Can you work these out from the drawing? Everything is in mm from the part's minimum corner. Give positions to 0.01 mm unless a question says otherwise; leave off trailing zeros. Write each loop counter-clockwise with the first axis right and the second up, starting at its lowest first coordinate (ties: lowest second). Pieces come first, ordered by that corner, then holes. Notation, with made-up numbers: (45, -37) - (89, -37) arc R19 ccw to (89, -7) - close; hole circle Ø5 at (-5.5, 59.5). An arc over 180 degrees is marked (long way). Use a Markdown table: item, result. Add a question column.
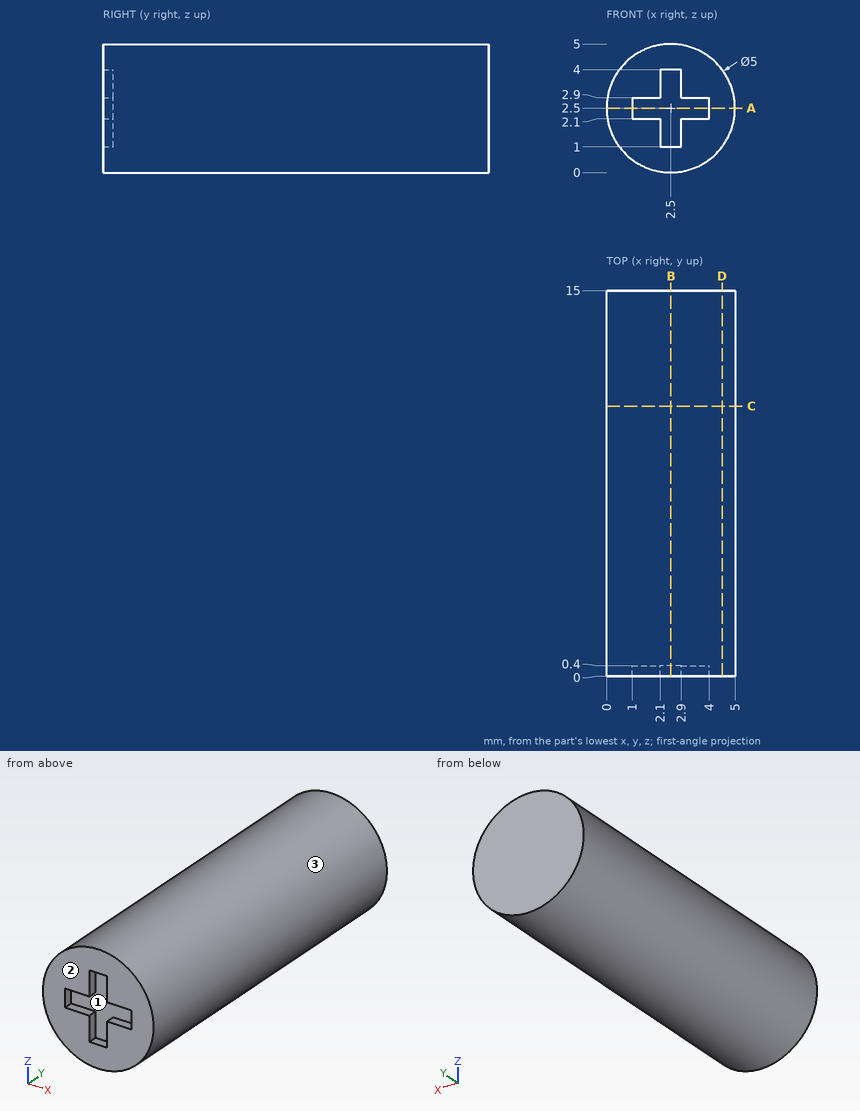
Q1. If I drill on probe 1 along Z at (x, y) = (0.55, 3); probe 2 along Z at (x, y) = (3.6, 11.25) (3 decimals); probe 3 along X at (y, z) = (5.5, 2.2), over which ranges is the centre line in solid material (lowest first)? Write a range as [from, to].
Q2. Suppose I cut it at A-A (z = 2.5). Please give me the cut outline in (x, y).
Q3. Suppose I cut it at C-C (y = 10.5). Please give me the cut outline in (x, z).
Q4. If we mould it in two halves opening along Z, with no side actions, what happens to the marked faces 1, 2 and 3? For each: released by +Z, released by -Z, zero draft, split by the parting line, or undercut.
Q5. Suppose I cut it at B-B (x = 2.5). Please give me the cut outline in (y, z), and give its area (3 significant figures).
Q6. Suppose I cut it at D-D (x = 4.5). Please give me the cut outline in (y, z).
Derived:
| question | item | result |
|---|---|---|
| 1 | probe 1 | [0.94, 4.06] |
| 1 | probe 2 | [0.255, 4.745] |
| 1 | probe 3 | [0.02, 4.98] |
| 2 | outline | (0, 0) - (1, 0) - (1, 0.4) - (4, 0.4) - (4, 0) - (5, 0) - (5, 15) - (0, 15) - close |
| 3 | outline | circle Ø5 at (2.5, 2.5) |
| 4 | face 1 | undercut |
| 4 | face 2 | zero draft |
| 4 | face 3 | split by the parting line |
| 5 | outline | (0, 0) - (15, 0) - (15, 5) - (0, 5) - (0, 4) - (0.4, 4) - (0.4, 1) - (0, 1) - close |
| 5 | area | 73.8 mm² |
| 6 | outline | (0, 1) - (15, 1) - (15, 4) - (0, 4) - close |
